Could you check a few things on this model? Use its own coordinates, in mm. A direction names the side the tool comes from. Coordinates: 2 decimals unless noted, no trailing zeros. Loops run counter-clockwise (first coordinate to the right, second up) from the corner with the lowest first, then second, coordinate; pieces in that order, holes last. Notation, with made-up numbers: (-25, 81) -> (1, 81) arc R9 ccw to (1, 98) -> close; hole circle Ø11 at (-11, 38.25). An arc over 180 degrees is marked (long way). One line per question, with ' | ' between items.
```python
from build123d import *

# Parameters (mm, degrees)
SKIZZE1_W                       = 18
SKIZZE1_H                       = 30
AUFSATZ_LINEAR_AUSTRAGEN1_DEPTH = 212.5
FASE1_SIZE                      = 12
FASE1_SIZE2                     = 44.784609691
F_7_0_7_DURCHMESSER_BOHRUNG1_D  = 7
SKIZZE4_W                       = 140
SKIZZE4_H                       = 5
SKIZZE4_W_2                     = 35
SKIZZE4_H_2                     = 2
SCHNITT_LINEAR_AUSTRAGEN1_DEPTH = 214.787862144
SCHNITT_LINEAR_AUSTRAGEN2_DEPTH = 214.787862144


with BuildPart() as part:
    # Skizze1 → Aufsatz-Linear austragen1 (new, symmetric)
    with BuildSketch(Plane(origin=(0, 0, 0), x_dir=(0, 0, -1), z_dir=(1, 0, 0))):
        Rectangle(SKIZZE1_W, SKIZZE1_H)
    extrude(amount=AUFSATZ_LINEAR_AUSTRAGEN1_DEPTH, both=True)

    # Fase1
    fase1_edges = [part.edges().sort_by_distance(p)[0] for p in [
        (-212.5, 0, 9),
    ]]
    fase1_side = [part.faces().sort_by_distance(p)[0] for p in [
        (-212.5, 0, 0),
    ]]
    chamfer(fase1_edges, length=FASE1_SIZE, length2=FASE1_SIZE2, reference=fase1_side[0])

    # Ø7.0 (7) Durchmesser Bohrung1 (through all)
    with Locations(Plane(origin=(0, 15, 0), x_dir=(1, 0, 0), z_dir=(0, 1, 0))):
        with Locations((-142.5, -1), (2.5, -1)):
            Hole(F_7_0_7_DURCHMESSER_BOHRUNG1_D / 2)

    # Skizze4 → Schnitt-Linear austragen1 (cut, through all)
    with BuildSketch(Plane.XY.offset(9)):
        with Locations((142.5, -12.5)):
            Rectangle(SKIZZE4_W, SKIZZE4_H)
        with Locations((-195, -14)):
            Rectangle(SKIZZE4_W_2, SKIZZE4_H_2)
    extrude(amount=-SCHNITT_LINEAR_AUSTRAGEN1_DEPTH, mode=Mode.SUBTRACT)

    # Skizze5 → Schnitt-Linear austragen2 (cut, through all)
    with BuildSketch(Plane.XY.offset(9)):
        Polygon((-178.5, 15), (-212.5, 15), (-212.5, -4.629909152), align=None)
    extrude(amount=-SCHNITT_LINEAR_AUSTRAGEN2_DEPTH, mode=Mode.SUBTRACT)


solid = part.part
```
Q1. Imagine slicing it at A-A on x = -142.5. Write out the boundary of the cut face in (y, z), plus the area to 3 significant figures.
Values follow:
outline: (-15, -9) -> (15, -9) -> (15, -2.5) -> (-15, -2.5) -> close; (-15, 4.5) -> (15, 4.5) -> (15, 9) -> (-15, 9) -> close | area: 330 mm2
Q2. We'd pull the mould along X, two halves only. Please class faces 4 (the face through (212.5, 3, 0)), 5 (the face through (-184.818, -0.21, 4.417)), 6 (the face through (-145.84, -0.21, -0.05)), 7 (the face through (-51, -15, 0)): released by +X, released by -X, zero draft, split by the parting line, or undercut.
Values follow:
face 4: released by +X | face 5: released by -X | face 6: undercut | face 7: zero draft
Q3. Imagine slicing it at D-D on x = 90. Write out the boundary of the cut face in (y, z).
Values follow:
outline: (-10, -9) -> (15, -9) -> (15, 9) -> (-10, 9) -> close
Q4. Imagine slicing it at B-B on z = 1. Write out the boundary of the cut face in (x, y), plus the area to 3 significant figures.
Values follow:
outline: (-197.57, -13) -> (-177.5, -13) -> (-177.5, -15) -> (-146, -15) -> (-146, 15) -> (-178.5, 15) -> (-197.57, 3.99) -> close; (-139, -15) -> (-1, -15) -> (-1, 15) -> (-139, 15) -> close; (6, -15) -> (72.5, -15) -> (72.5, -10) -> (212.5, -10) -> (212.5, 15) -> (6, 15) -> close | area: 11,000 mm2
Q5. Imagine slicing it at C-C on y = 4. Write out the boundary of the cut face in (x, z), plus the area to 3 significant figures.
Values follow:
outline: (-197.55, -9) -> (212.5, -9) -> (212.5, 9) -> (-167.72, 9) -> (-197.55, 1.01) -> close; hole circle Ø7 at (-142.5, 1); hole circle Ø7 at (2.5, 1) | area: 7,180 mm2
Q6. Please list where these lines run through material, in increasing order: L1, parallel to Z at x = -142, y = -4; L2, parallel to Y at x = 134, z = 3.75; L3, parallel to X at y = 1, z = -5.75. Write a range as [from, to].
Values follow:
L1: z = [-9, -2.46], [4.46, 9] | L2: y = [-10, 15] | L3: x = [-202.75, 212.5]
Q7. For faces 1 (the face through (142, -10, 0)), 2 (the face through (-191, -13, -3)), 3 (the face through (3, 0, -9)), which set-ups out of +Z, -Z, +X, -X, +Y, -Y let a thin tool reach every point of the face, with its end or its side?
Values follow:
face 1: +Z, -Z, +X, -Y | face 2: +Z, -Z, -X, -Y | face 3: -Z, +X, -X, +Y, -Y
Q8. For pin 1 (4 mm diameter, centred on y = -13, z = 2, fed in from +X); pin 2 (3 mm diameter, centred on x = -141.5, z = 1, fed in from +Y); pin 3 (5.5 mm diameter, centred on x = 129.5, z = 1.5, fed in from -Y); pin 4 (4.5 mm diameter, centred on x = -196.5, z = -5, fed in from -Y), each with a flat end and sliding along its axis, tell me the tip position at first contact or that it passes through.
Values follow:
pin 1: stops at x = 72.5 | pin 2: passes through | pin 3: stops at y = -10 | pin 4: stops at y = -13
